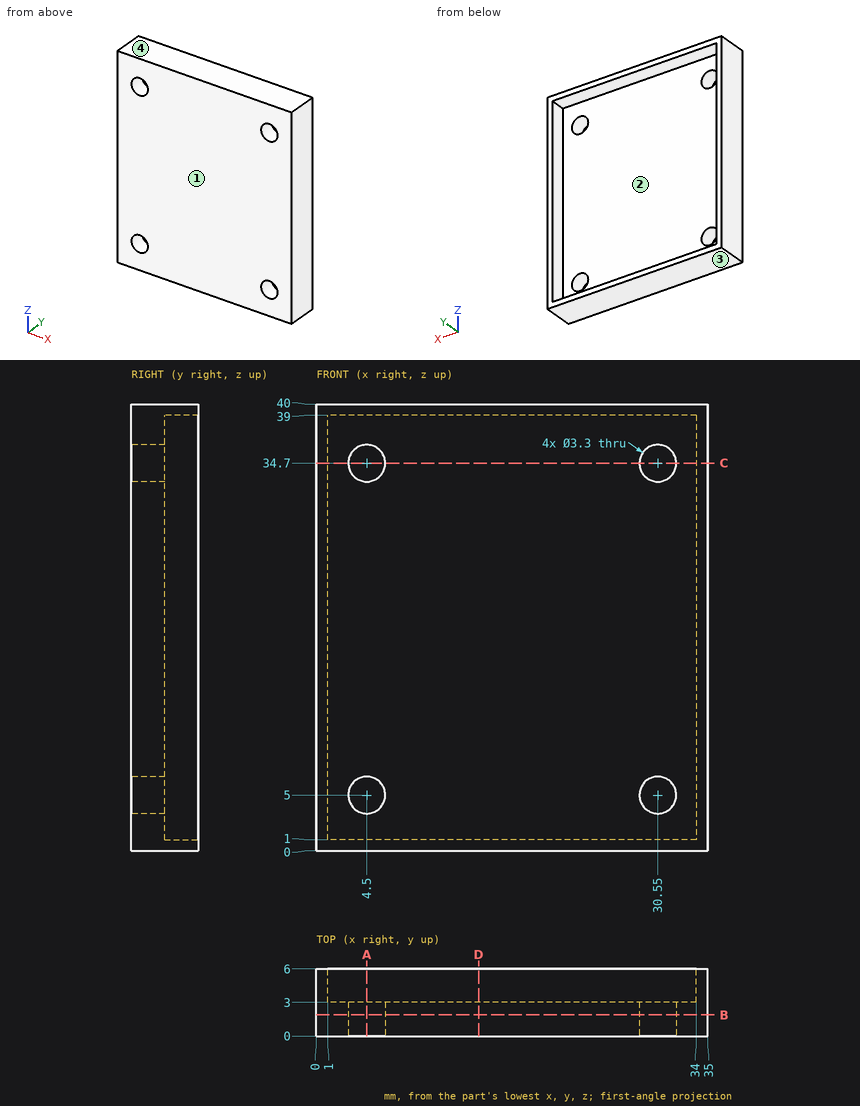
The figure shows three views and two pictorial views of one solid part (mm, origin at its lowest corner). Answer the questions. Round coordinates to 2 decimals unless told otherwise and drop trailing zeros. Order: outer loops, then holes, each group sorted by start corner. A loop starts at its lowest first (then second) coordinate and runs counter-clockwise, first axis right, second up. Notation, with made-up numbers: (79, 16.25) -> (103, 16.25) arc R18 ccw to (103, 51.25) -> close; hole circle Ø7 at (62, 9.5). An arc over 180 degrees is marked (long way). Put each result on its own line as item: value.
Q1. Section B-B, the plane y = 1.9 is taken. Write down the section's boundary in (x, z), and give its area (3 significant figures).
Results list:
outline: (0, 0) -> (35, 0) -> (35, 40) -> (0, 40) -> close; hole circle Ø3.3 at (4.5, 5); hole circle Ø3.3 at (4.5, 34.7); hole circle Ø3.3 at (30.55, 5); hole circle Ø3.3 at (30.55, 34.7)
area: 1,370 mm^2
Q2. Section D-D, the plane x = 14.5 is taken. Write down the section's boundary in (y, z).
Results list:
outline: (0, 0) -> (6, 0) -> (6, 1) -> (3, 1) -> (3, 39) -> (6, 39) -> (6, 40) -> (0, 40) -> close
Q3. Consider line 1 along Z through (x, y) = (30.55, 2); line 2 along X through (y, z) = (1.95, 34.7); line 3 along X through (y, z) = (4.3, 36). Determine where each line is inside the solid, lowest interval first.
Results list:
line 1: 0 to 3.35, 6.65 to 33.05, 36.35 to 40
line 2: 0 to 2.85, 6.15 to 28.9, 32.2 to 35
line 3: 0 to 1, 34 to 35
Q4. Determine the mould class of the marked faces 1, 2, 3 and 4 for opening direction Z: pulls with the +Z half, pulls with the -Z half, needs draft (parallel to the pull), parting line crosses it, or undercut.
Results list:
face 1: needs draft
face 2: undercut
face 3: pulls with the -Z half
face 4: pulls with the +Z half
Q5. This flat-tipped pin is pushed along its axis until it touches: P1, Ø2, axis at x = 13.5, z = 14, coming from the +Y side. Where does it stop, or does it pass through?
Results list:
P1: y = 3
Q6. Section A-A, the plane x = 4.5 is taken. Write down the section's boundary in (y, z), and give its area (3 significant figures).
Results list:
outline: (0, 0) -> (6, 0) -> (6, 1) -> (3, 1) -> (3, 3.35) -> (0, 3.35) -> close; (0, 6.65) -> (3, 6.65) -> (3, 33.05) -> (0, 33.05) -> close; (0, 36.35) -> (3, 36.35) -> (3, 39) -> (6, 39) -> (6, 40) -> (0, 40) -> close
area: 106 mm^2
Q7. Section C-C, the plane z = 34.7 is taken. Write down the section's boundary in (x, y).
Results list:
outline: (0, 0) -> (2.85, 0) -> (2.85, 3) -> (1, 3) -> (1, 6) -> (0, 6) -> close; (6.15, 0) -> (28.9, 0) -> (28.9, 3) -> (6.15, 3) -> close; (32.2, 0) -> (35, 0) -> (35, 6) -> (34, 6) -> (34, 3) -> (32.2, 3) -> close
